Geometry: see drawing. Coordinates: mm, zero at the bounding-box minimum. A direction names the side the tool comes from. Coordinates: 2 decimals unless noted, no trailing zeros. Write each loop counter-clockwise with the first axis right and the second up, starting at its lowest first coordinate (ties: lowest second). Pieces come first, ordered by that corner, then holes. Notation, with made-up numbers: M -39.75,-10.75 L 7.25,-10.75 A23 cw 7.25,27.25 Z; hole C 7,13 d11. An arc over 180 degrees is marked long. Write item = value, one per line. Start each with the question number.
1. Pin query (flat end, axial travel): pin 1 Ø5 at (x, z) = (11, 7.52) entering from +Y; pin 2 Ø4 at (x, y) = (3, 11) entering from -Z; pin 3 Ø3 at (x, y) = (8, 5) entering from +Z; pin 4 Ø2.5 at (x, y) = (11, 3) entering from +Z. Return the tip coordinate at first contact, or that it passes through.
2. Pull-direction query (X, two-part tool) for the marked faces 1, 2 and 3; classes: pulls with the +X half, pulls with the -X half, needs draft (parallel to the pull), parting line crosses it, or undercut.
3. Section query A-A (y = 11). Output: boundary loops of the cut face in (x, z) (3 decimals), then the cut area to 3 significant figures.
4. Section query C-C (z = 4.25). Output: boundary loops of the cut face in (x, y) (3 decimals).
5. Line query: line 1 along Z through (x, y) = (9, 4.5); line 2 along Y through (x, z) = (13.25, 8.25) (1 decimal); line 3 along X through (y, z) = (11.75, 10.5) (1 decimal). Output: solid intervals per line, ascending.
6. Section query B-B (x = 11). Output: boundary loops of the cut face in (y, z) (3 decimals), then the cut area to 3 significant figures.
7. Section query D-D (y = 19). Output: boundary loops of the cut face in (x, z), then the cut area to 3 significant figures.
8. Access query for the marked faces 4, 5 and 6. Directions: +Z, -Z, +X, -X, +Y, -Y. A direction counts if a zero-diameter tool reaches every point of the face in a straight line with its end or side. Return the directions, or none.
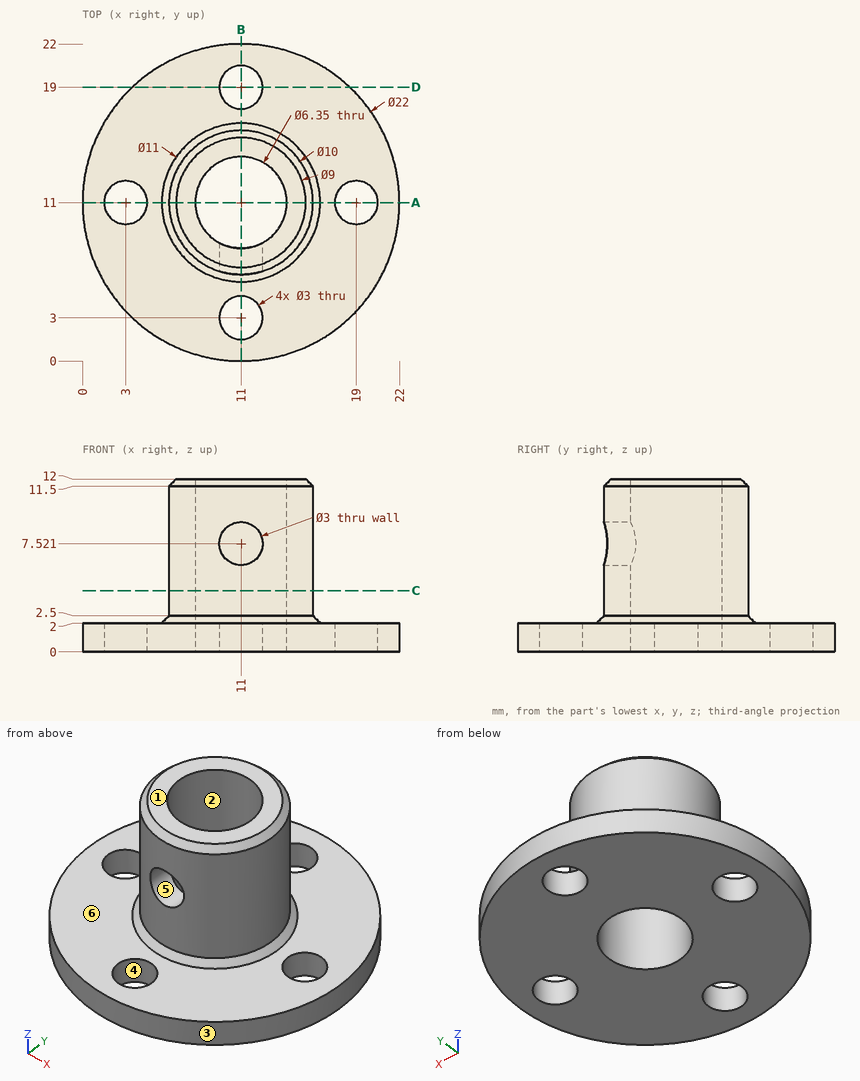
Results are:
q1.pin_1 = 16
q1.pin_2 = 0
q1.pin_3 = 2.29
q1.pin_4 = through
q2.face_1 = needs draft
q2.face_2 = undercut
q2.face_3 = parting line crosses it
q3.outline = M 0,0 L 1.5,0 L 1.5,2 L 0,2 Z; M 4.5,0 L 7.825,0 L 7.825,12 L 6.5,12 L 6,11.5 L 6,2.5 L 5.5,2 L 4.5,2 Z; M 14.175,0 L 17.5,0 L 17.5,2 L 16.5,2 L 16,2.5 L 16,11.5 L 15.5,12 L 14.175,12 Z; M 20.5,0 L 22,0 L 22,2 L 20.5,2 Z
q3.area = 55.8 mm^2
q4.outline = C 11,11 d10; hole C 11,11 d6.35
q5.line_1 = 0 to 2
q5.line_2 = 6.5 to 8.8, 13.2 to 15.5
q5.line_3 = 6.1 to 7.9, 14.1 to 15.9
q6.outline = M 0,0 L 1.5,0 L 1.5,2 L 0,2 Z; M 4.5,0 L 7.825,0 L 7.825,6.021 L 6,6.021 L 6,2.5 L 5.5,2 L 4.5,2 Z; M 6,9.021 L 7.825,9.021 L 7.825,12 L 6.5,12 L 6,11.5 Z; M 14.175,0 L 17.5,0 L 17.5,2 L 16.5,2 L 16,2.5 L 16,11.5 L 15.5,12 L 14.175,12 Z; M 20.5,0 L 22,0 L 22,2 L 20.5,2 Z
q6.area = 50.3 mm^2
q7.outline = M 3.45,0 L 9.5,0 L 9.5,2 L 3.45,2 Z; M 12.5,0 L 18.55,0 L 18.55,2 L 12.5,2 Z
q7.area = 24.2 mm^2
q8.face_4 = +Z, -Z
q8.face_5 = -Y
q8.face_6 = +Z
